Verification items for the finished model (mm, model axes). A direction names the side the tool comes from. Give positions to 0.01 mm unless a question says otherwise; leave off trailing zeros. Loops run counter-clockwise (first coordinate to the right, second up) from the corner with the lowest first, then second, coordinate; pieces in that order, holes last. Notation, with made-up numbers: M 77,-21 L 89,-21 A12 cw 89,-9 Z; hole C 86,64 d1. An arc over 180 degrees is marked long. Use CSV: the item, a comma, the result in double quotes.
from build123d import *

# Parameters (mm, degrees)
BOSS_EXTRUDE1_DEPTH = 5.08
BOSS_EXTRUDE2_DEPTH = 1.651
SKETCH4_R           = 1.03378
CUT_EXTRUDE1_DEPTH  = 3.175


with BuildPart() as part:
    # Sketch2 → Boss-Extrude1 (new body)
    with BuildSketch(Plane.XY):
        with BuildLine():
            ThreePointArc((-81.80598839, 6.218522937), (-75.819, 0), (-81.80598839, -6.218522937))
            ThreePointArc((-81.80598839, -6.218522937), (-82.042, 0), (-81.80598839, 6.218522937))
        make_face()
    extrude(amount=BOSS_EXTRUDE1_DEPTH)

    # Sketch3 → Boss-Extrude2 (add)
    with BuildSketch(Plane.XY.offset(5.08)):
        with BuildLine():
            Line((-81.80598839, 6.218522937), (-74.279907283, 5.53037832))
            ThreePointArc((-74.279907283, 5.53037832), (-74.4855, 0), (-74.279907283, -5.53037832))
            Line((-74.279907283, -5.53037832), (-81.80598839, -6.218522937))
            ThreePointArc((-81.80598839, -6.218522937), (-82.042, 0), (-81.80598839, 6.218522937))
        make_face()
    extrude(amount=BOSS_EXTRUDE2_DEPTH)

    # Sketch4 → Cut-Extrude1 (cut)
    with BuildSketch(Plane.ZY.offset(82.042)):
        with Locations((3.683, 0)):
            Circle(SKETCH4_R)
    extrude(amount=-CUT_EXTRUDE1_DEPTH, mode=Mode.SUBTRACT)


solid = part.part
(1) Tool access check on faces 5 (the flat face through (-78, 0, 6.731)), 6 (the cylindrical face through (-80.48, 0.31, 4.67)), 7 (the flat face through (-75, 0, 5.08)). Record the directions out of +Z, -Z, +X, -X, +Y, -Y that give a thin tool (end or side, any length) a straight path to the whole face; none if there is none.
Calculated:
face 5,"+Z, +X, -X, +Y, -Y"
face 6,"-X"
face 7,"-Z, +X"
(2) Section check C-C on z = 5.75. Record the cut outline in (x, y).
Calculated:
outline,"M -81.81,-6.22 L -74.28,-5.53 A74.49 cw -74.28,5.53 L -81.81,6.22 A82.04 ccw Z"
(3) Depth check by flat-ended pin: pin 1 Ø4 at (x, z) = (-79.5, 2) entering from +Y. Enter the tip coordinate at first touch or a pass-through.
Calculated:
pin 1,"stops at y = 6.2"
(4) Mould release check, pull along Y, two halves, no side actions. Record for faces 1 (the flat face through (-78.1, 5.88, 5.89)), 2 (the flat face through (-80, 0, 0)), 3 (the cylindrical face through (-75.82, 0.13, 2.5)), 4 (the cylindrical face through (-74.485, 0.077, 5.894)): released by +Y, released by -Y, zero draft, split by the parting line, or undercut.
Calculated:
face 1,"released by +Y"
face 2,"zero draft"
face 3,"split by the parting line"
face 4,"undercut"
(5) Scan lines: L1, parallel to Z at x = -81.15, y = 0; L2, parallel to Y at x = -79.75, z = 4; L3, parallel to Z at x = -74.75, y = 4. Record each from-to range of solid material in increasing order. Write a range as from..to.
Calculated:
L1,"z = 0..2.65, 4.72..6.73"
L2,"y = -5.79..-0.98, 0.98..5.79"
L3,"z = 5.08..6.73"
(6) Section check A-A on y = 0. Record the cut outline in (x, z).
Calculated:
outline,"M -82.04,0 L -75.82,0 L -75.82,5.08 L -74.49,5.08 L -74.49,6.73 L -82.04,6.73 L -82.04,4.72 L -78.87,4.72 L -78.87,2.65 L -82.04,2.65 Z"
(7) Section check D-D on x = -76.5. Record the cut outline in (y, z).
Calculated:
outline,"M -5.73,5.08 L -2.83,5.08 L -2.83,0 L 2.83,0 L 2.83,5.08 L 5.73,5.08 L 5.73,6.73 L -5.73,6.73 Z"
(8) Section check B-B on x = -79.75. Record the cut outline in (y, z).
Calculated:
outline,"M -6.03,5.08 L -5.79,5.08 L -5.79,0 L 5.79,0 L 5.79,5.08 L 6.03,5.08 L 6.03,6.73 L -6.03,6.73 Z; hole C 0,3.68 d2.07"
